Input: dimensioned drawing with shaded views. Units: mm. Origin: part minimum x, y, z. Coordinates: 2 decimals unless noted, no trailing zeros. Loops run counter-clockwise (first coordinate to the right, second up) from the corner with the lowest first, then second, coordinate; pieces in that order, holes last. Notation, with made-up numbers: (14.25, -36.75) - (46.25, -36.75) arc R22 cw to (46.25, -7.75) - close; hole circle Ø6 at (9.25, 70.25). An arc over 180 degrees is marked (long way). Put each result on its own line as item: value. Start each with the question number.
1) Section A-A on z = 383.5. Output: boundary loops of the cut face in (x, y).
2) Contact query for flat-ended pins moving along their axis: pin 1 Ø6.5 at (y, z) = (7.5, 153.5) entering from +X; pin 2 Ø6.5 at (x, y) = (362, 4.5) entering from +Z; pin 3 Ø4 at (x, y) = (361.5, 7.5) entering from -Z. Output: stop coordinate, or through.
3) Draft query along X for the marked faces 1, 2, 3 and 4. Return one class per face: +X half, -X half, draft (parallel to the pull), parting line (faces both ways), or undercut.
4) Material intervals for line 1 along X through (y, z) = (19, 291.5); line 2 along Y through (x, z) = (75, 268.5); line 3 along Y through (x, z) = (301, 329), sorted ascending. Write a range as from..to.
5) Section C-C on z = 181. Output: boundary loops of the cut face in (x, y), and give its area (3 significant figures).
6) Section B-B on x = 395. Output: boundary loops of the cut face in (y, z).
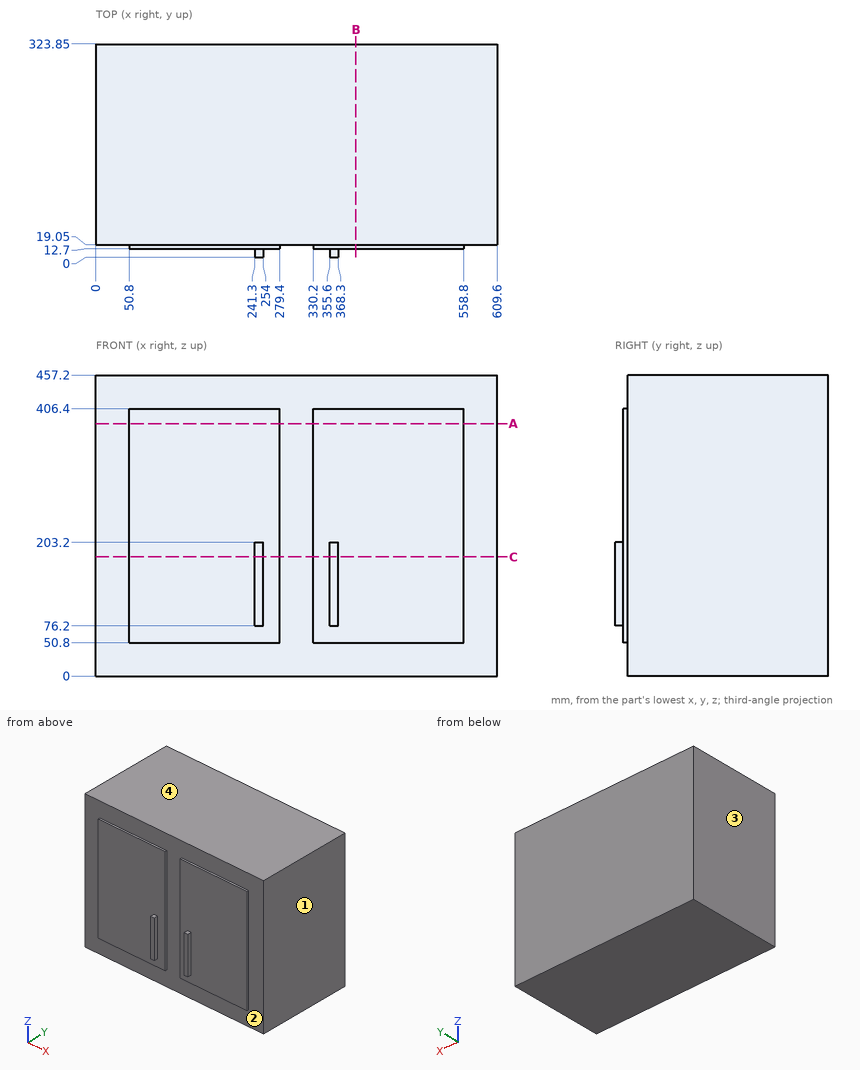
Answer block:
1. outline: (0, 19.05) - (50.8, 19.05) - (50.8, 12.7) - (279.4, 12.7) - (279.4, 19.05) - (330.2, 19.05) - (330.2, 12.7) - (558.8, 12.7) - (558.8, 19.05) - (609.6, 19.05) - (609.6, 323.85) - (0, 323.85) - close
2. pin 1: stops at x = 368.3
2. pin 2: stops at z = 203.2
2. pin 3: stops at z = 76.2
3. face 1: +X half
3. face 2: undercut
3. face 3: -X half
3. face 4: draft
4. line 1: x = 50.8..279.4, 330.2..558.8
4. line 2: y = 12.7..323.85
4. line 3: y = 19.05..323.85
5. outline: (0, 19.05) - (50.8, 19.05) - (50.8, 12.7) - (241.3, 12.7) - (241.3, 0) - (254, 0) - (254, 12.7) - (279.4, 12.7) - (279.4, 19.05) - (330.2, 19.05) - (330.2, 12.7) - (355.6, 12.7) - (355.6, 0) - (368.3, 0) - (368.3, 12.7) - (558.8, 12.7) - (558.8, 19.05) - (609.6, 19.05) - (609.6, 323.85) - (0, 323.85) - close
5. area: 189,000 mm²
6. outline: (12.7, 50.8) - (19.05, 50.8) - (19.05, 0) - (323.85, 0) - (323.85, 457.2) - (19.05, 457.2) - (19.05, 406.4) - (12.7, 406.4) - close
